Geometry check sheet. Reference: drawing and pictorial views, mm from the part's lowest x, y, z. A direction names the side the tool comes from. Give positions to 0.01 mm unless a question says otherwise; leave off trailing zeros. Write each loop counter-clockwise with the first axis right and the second up, starting at its lowest first coordinate (ties: lowest second). Pieces come first, ordered by that corner, then holes. Notation, with made-up numbers: (-22, -30.75) -> (-15, -30.75) arc R7 cw to (-15, -21.75) -> close; hole circle Ø10 at (47.25, -36). An arc over 180 degrees is marked (long way). Return JSON: item names as keys, results as strings.
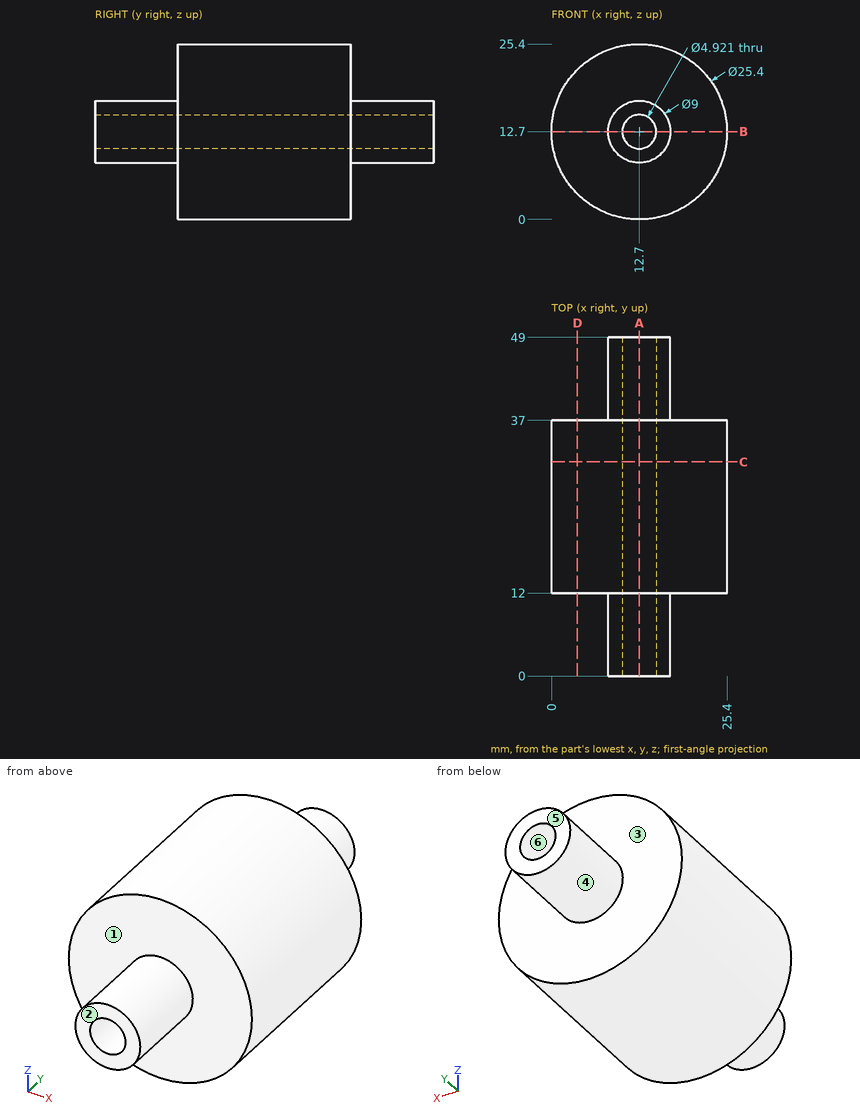
(1) Thickness scan on L1, parallel to X at y = 19, z = 12.7; L2, parallel to X at y = 11, z = 12.7; L3, parallel to Y at x = 10.5, z = 21.5. Record the ranges inside material, lowest first.
Reply:
{"L1": "0 to 10.24, 15.16 to 25.4", "L2": "8.2 to 10.24, 15.16 to 17.2", "L3": "12 to 37"}
(2) Set-up check for the marked faces 1, 2 and 3: record each of +Z, -Z, +X, -X, +Y, -Y from which the full face is reachable in a straight line by a thin tool's end or side.
Reply:
{"face 1": "-Y", "face 2": "+Z, -Z, +X, -X, -Y", "face 3": "+Y"}
(3) Cross-section at B-B on z = 12.7. Enter the section's corners in (x, y).
Reply:
{"outline": "(0, 12) -> (8.2, 12) -> (8.2, 0) -> (10.24, 0) -> (10.24, 49) -> (8.2, 49) -> (8.2, 37) -> (0, 37) -> close; (15.16, 0) -> (17.2, 0) -> (17.2, 12) -> (25.4, 12) -> (25.4, 37) -> (17.2, 37) -> (17.2, 49) -> (15.16, 49) -> close"}
(4) Cross-section at A-A on x = 12.7. Enter the section's corners in (y, z).
Reply:
{"outline": "(0, 8.2) -> (12, 8.2) -> (12, 0) -> (37, 0) -> (37, 8.2) -> (49, 8.2) -> (49, 10.24) -> (0, 10.24) -> close; (0, 15.16) -> (49, 15.16) -> (49, 17.2) -> (37, 17.2) -> (37, 25.4) -> (12, 25.4) -> (12, 17.2) -> (0, 17.2) -> close"}
(5) Depth check by flat-ended pin: pin 1 Ø12 at (y, z) = (40, 6) entering from +X; pin 2 Ø12 at (y, z) = (39, 6.5) entering from -X; pin 3 Ø12 at (x, y) = (3, 32) entering from +Z; pin 4 Ø4.5 at (x, z) = (12.7, 12.7) entering from -Y. Enter the tip coordinate at first touch or a pass-through.
Reply:
{"pin 1": "x = 25.31", "pin 2": "x = 0.01", "pin 3": "z = 24.85", "pin 4": "through"}
(6) Release check for a two-part mould opening along Z. For the marked faces 4, 5 and 6 record: pulls with the +Z half, pulls with the -Z half, needs draft (parallel to the pull), parting line crosses it, or undercut.
Reply:
{"face 4": "parting line crosses it", "face 5": "needs draft", "face 6": "undercut"}
(7) Cross-section at C-C on y = 31. Enter the section's corners in (x, z), then the cut area to 3 significant figures.
Reply:
{"outline": "circle Ø25.4 at (12.7, 12.7); hole circle Ø4.92 at (12.7, 12.7)", "area": "488 mm^2"}
(8) Cross-section at D-D on x = 3.75. Enter the section's corners in (y, z).
Reply:
{"outline": "(12, 3.69) -> (37, 3.69) -> (37, 21.71) -> (12, 21.71) -> close"}
